The listing builds one solid part. Answer for the finished solid, in the listing's coordinates (mm). Give positions to 0.01 mm unless a question says otherwise; leave off trailing zeros. Loops run counter-clockwise (first coordinate to the right, second up) from the corner with the lowest first, then second, coordinate; pieces in that order, holes last. Notation, with made-up numbers: (47, 8.5) - (59, 8.5) arc R20 cw to (59, 23.5) - close; hole circle Ø3 at (71, 25). An arc over 180 degrees is marked (long way). Write each question's results on one line, items separated by ' | '.
from build123d import *

# Parameters (mm, degrees)
SKETCH1_W            = 74.07
SKETCH1_H            = 50.8
BOSS_EXTRUDE1_DEPTH  = 6.35
FILLET1_R            = 10
M5_CLEARANCE_HOLE1_D = 5.5
BOSS_EXTRUDE2_DEPTH  = 6.35
SKETCH5_R            = 11.25
CUT_EXTRUDE1_DEPTH   = 7.35
FILLET2_R            = 10
FILLET3_R            = 22.5


with BuildPart() as part:
    # Sketch1 → Boss-Extrude1 (new body)
    with BuildSketch(Plane.XY):
        Rectangle(SKETCH1_W, SKETCH1_H)
    extrude(amount=BOSS_EXTRUDE1_DEPTH)

    # Fillet1
    fillet1_edges = [part.edges().sort_by_distance(p)[0] for p in [
        (-37.035, 25.4, 3.175),
        (37.035, 25.4, 3.175),
        (37.035, -25.4, 3.175),
        (-37.035, -25.4, 3.175),
    ]]
    fillet(fillet1_edges, radius=FILLET1_R)

    # M5 Clearance Hole1 (through all)
    with Locations(Plane.XY.offset(6.35)):
        with Locations((-26.465, 12.7), (-26.465, -12.7), (-1.065, -12.7), (-1.065, 12.7), (24.335, 12.7), (24.335, -12.7)):
            Hole(M5_CLEARANCE_HOLE1_D / 2)

    # Sketch4 → Boss-Extrude2 (add)
    with BuildSketch(Plane.XY.offset(6.35)):
        Polygon((37.035, -15.4), (37.035, -70.4), (-37.035, -70.4), (-37.035, -15.4), (-27.035, -25.4), (27.035, -25.4), align=None)
    extrude(amount=-BOSS_EXTRUDE2_DEPTH)

    # Sketch5 → Cut-Extrude1 (cut, through all)
    with BuildSketch(Plane.XY.offset(6.35)):
        with Locations((14.535, -47.9)):
            Circle(SKETCH5_R)
    extrude(amount=-CUT_EXTRUDE1_DEPTH, mode=Mode.SUBTRACT)

    # Fillet2
    fillet2_edges = [part.edges().sort_by_distance(p)[0] for p in [
        (-37.035, -70.4, 3.175),
    ]]
    fillet(fillet2_edges, radius=FILLET2_R)

    # Fillet3
    fillet3_edges = [part.edges().sort_by_distance(p)[0] for p in [
        (37.035, -70.4, 3.175),
    ]]
    fillet(fillet3_edges, radius=FILLET3_R)


solid = part.part
Item 1: Find the intervals of material crossed by line 1 along Y through (x, z) = (-1, 4); line 2 along Y through (x, z) = (1, 2.25); line 3 along Y through (x, z) = (5, 2), in increasing order. Write a range as [from, to].
Values found:
line 1: y = [-70.4, -15.45], [-9.95, 9.95], [15.45, 25.4] | line 2: y = [-70.4, -14.52], [-10.88, 10.88], [14.52, 25.4] | line 3: y = [-70.4, -53.87], [-41.93, 25.4]
Item 2: A cutting plane is placed at A-A, the plane y = -12.7. Determine the outline of the cut face in (x, z) (3 decimals), plus the area to 3 significant figures.
Values found:
outline: (-37.035, 0) - (-29.215, 0) - (-29.215, 6.35) - (-37.035, 6.35) - close; (-23.715, 0) - (-3.815, 0) - (-3.815, 6.35) - (-23.715, 6.35) - close; (1.685, 0) - (21.585, 0) - (21.585, 6.35) - (1.685, 6.35) - close; (27.085, 0) - (37.035, 0) - (37.035, 6.35) - (27.085, 6.35) - close | area: 366 mm²
Item 3: A cutting plane is placed at B-B, the plane x = 24.5. Determine the outline of the cut face in (y, z), plus the area to 3 significant figures.
Values found:
outline: (-68.07, 0) - (-53.12, 0) - (-53.12, 6.35) - (-68.07, 6.35) - close; (-42.68, 0) - (-15.45, 0) - (-15.45, 6.35) - (-42.68, 6.35) - close; (-9.95, 0) - (9.95, 0) - (9.95, 6.35) - (-9.95, 6.35) - close; (15.45, 0) - (25.4, 0) - (25.4, 6.35) - (15.45, 6.35) - close | area: 458 mm²
Item 4: For a pull along Y with two mould halves and no side action, classify faces 1 (the face through (0, 25.4, 3)), 2 (the face through (12.096, -58.882, 3.219)), 3 (the face through (30.269, -63.984, 3.131)) as released by +Y, released by -Y, zero draft, split by the parting line, or undercut.
Values found:
face 1: released by +Y | face 2: undercut | face 3: released by -Y
Item 5: A cutting plane is placed at D-D, the plane y = -57. Determine the outline of the cut face in (x, z) (3 decimals).
Values found:
outline: (-37.035, 0) - (7.92, 0) - (7.92, 6.35) - (-37.035, 6.35) - close; (21.15, 0) - (35.113, 0) - (35.113, 6.35) - (21.15, 6.35) - close
Item 6: A cutting plane is placed at C-C, the plane z = 4. Determine the outline of the cut face in (x, y) (3 decimals).
Values found:
outline: (-37.035, -60.4) arc R10 ccw to (-27.035, -70.4) - (14.535, -70.4) arc R22.5 ccw to (37.035, -47.9) - (37.035, 15.4) arc R10 ccw to (27.035, 25.4) - (-27.035, 25.4) arc R10 ccw to (-37.035, 15.4) - close; hole circle Ø5.5 at (-26.465, -12.7); hole circle Ø5.5 at (-26.465, 12.7); hole circle Ø5.5 at (-1.065, -12.7); hole circle Ø5.5 at (-1.065, 12.7); hole circle Ø22.5 at (14.535, -47.9); hole circle Ø5.5 at (24.335, -12.7); hole circle Ø5.5 at (24.335, 12.7)
